```python
from build123d import *

# Parameters (mm, degrees)
SKETCH1_R           = 10.5
BOSS_EXTRUDE1_DEPTH = 16.5
SKETCH2_R           = 7.5
CUT_EXTRUDE1_DEPTH  = 9
SKETCH15_R          = 0.5
CUT_EXTRUDE10_DEPTH = 3
CIRPATTERN1_COUNT   = 4
SKETCH11_R          = 2.75
CUT_EXTRUDE6_DEPTH  = 23.19797288
SKETCH13_W          = 5
SKETCH13_H          = 21
CUT_EXTRUDE8_DEPTH  = 23.197973064
SKETCH14_R          = 0.5
CUT_EXTRUDE9_DEPTH  = 2


with BuildPart() as part:
    # Sketch1 → Boss-Extrude1 (new body)
    with BuildSketch(Plane.XY):
        Circle(SKETCH1_R)
    extrude(amount=BOSS_EXTRUDE1_DEPTH)

    # Sketch2 → Cut-Extrude1 (cut)
    with BuildSketch(Plane.XY.offset(16.5)):
        Circle(SKETCH2_R)
    extrude(amount=-CUT_EXTRUDE1_DEPTH, mode=Mode.SUBTRACT)

    # Sketch15 → Cut-Extrude10 (cut)
    with BuildSketch(Plane.XY.offset(16.5)):
        with Locations((6.363961031, 6.363961031)):
            Circle(SKETCH15_R)
    cut_extrude10 = extrude(amount=-CUT_EXTRUDE10_DEPTH, mode=Mode.SUBTRACT)

    # CirPattern1: Cut-Extrude10 ×4 about axis
    cirpattern1_axis = Axis((0, 0, 0), (0, 0, 1))
    for i in range(1, CIRPATTERN1_COUNT):
        add(cut_extrude10.rotate(cirpattern1_axis, i * 360 / CIRPATTERN1_COUNT), mode=Mode.SUBTRACT)

    # Sketch9 → Cut-Revolve1 (revolve, cut)
    with BuildSketch(Plane(origin=(0, 0, 0), x_dir=(0, 0, -1), z_dir=(1, 0, 0)), mode=Mode.PRIVATE) as cut_revolve1_sk:
        Polygon((-5, 0), (-5, 7.5), (-2.5, 7.5), (-2.5, 5.5), (0, 5.5), (0, 0), align=None)
    revolve(cut_revolve1_sk.sketch.rotate(Axis((0, 0, 0), (0, 0, 1)), 90), axis=Axis((0, 0, 0), (0, 0, 1)), mode=Mode.SUBTRACT)

    # Sketch11 → Cut-Extrude6 (cut, through all)
    with BuildSketch(Plane(origin=(0, 0, 0), x_dir=(0, 0, -1), z_dir=(1, 0, 0))):
        with Locations((-11.75, 0)):
            Circle(SKETCH11_R)
    extrude(amount=-CUT_EXTRUDE6_DEPTH, mode=Mode.SUBTRACT)

    # Sketch13 → Cut-Extrude8 (cut, through all)
    with BuildSketch(Plane(origin=(0, 0, 0), x_dir=(0, 0, -1), z_dir=(1, 0, 0))):
        with Locations((-2.5, 0)):
            Rectangle(SKETCH13_W, SKETCH13_H)
    extrude(amount=-CUT_EXTRUDE8_DEPTH, mode=Mode.SUBTRACT)

    # Sketch14 → Cut-Extrude9 (cut)
    with BuildSketch(Plane.ZY):
        with Locations((2.5, 9)):
            Circle(SKETCH14_R)
    cut_extrude9 = extrude(amount=-CUT_EXTRUDE9_DEPTH, mode=Mode.SUBTRACT)

    # Mirror1: Cut-Extrude9 across plane
    add(cut_extrude9.mirror(Plane.ZX), mode=Mode.SUBTRACT)


solid = part.part
```
Geometry: final body of the model. Coordinates: model frame, mm. A direction names the side the tool comes from. Round coordinates to 2 decimals unless told otherwise and drop trailing zeros. Order: outer loops, then holes, each group sorted by start corner. A loop starts at its lowest first (then second) coordinate and runs counter-clockwise, first axis right, second up. Notation, with made-up numbers: (-4.75, 26) -> (4.25, 26) arc R24 cw to (4.25, 59) -> close; hole circle Ø5 at (42.25, -1). An arc over 180 degrees is marked (long way). Use one line per item in the form item = value.
(1) Access query for faces 4 (the face through (2, -9, 2.5)), 5 (the face through (0, 8.59, 1.98)), 6 (the face through (5, -7, 16.5)), 7 (the face through (6, 0, 0)), 8 (the face through (6.4, -6.4, 13.5)). Directions: +Z, -Z, +X, -X, +Y, -Y. A direction counts if a zero-diameter tool reaches every point of the face in a straight line with its end or side. Return the directions, or none.
Results list:
face_4 = -X
face_5 = -Z, -X, +Y, -Y
face_6 = +Z, +X, -X, +Y, -Y
face_7 = -Z, +X, -X, +Y, -Y
face_8 = +Z
(2) First-contact query: pin 1 Ø3 at (y, z) = (-6.5, 5.5) entering from -X; pin 2 Ø1 at (x, z) = (-3.5, 14) entering from -Y; pin 3 Ø0.5 at (y, z) = (9, 2.5) entering from -X. Flat tips, straight axial feed; report the tip coordinate or a pass-through.
Results list:
pin_1 = -9.23
pin_2 = -10.06
pin_3 = 2
(3) Draft query along Z for faces 1 (the face through (1, -9, 2)), 2 (the face through (-6.4, 6.4, 13.5)), 3 (the face through (6.841, 6.514, 15.021)). Return one class per face: pulls with the +Z half, pulls with the -Z half, needs draft (parallel to the pull), parting line crosses it, or undercut.
Results list:
face_1 = undercut
face_2 = pulls with the +Z half
face_3 = needs draft
(4) Section D-D on z = 5.5. Return loops of the section in (x, y), and give its area (3 significant figures).
Results list:
outline = circle Ø21 at (0, 0)
area = 346 mm^2
(5) Section B-B on x = 1.5. Return loops of the section in (y, z), and give its area (3 significant figures).
Results list:
outline = (-10.39, 0) -> (-5.29, 0) -> (-5.29, 2.5) -> (-7.35, 2.5) -> (-7.35, 5) -> (7.35, 5) -> (7.35, 2.5) -> (5.29, 2.5) -> (5.29, 0) -> (10.39, 0) -> (10.39, 16.5) -> (7.35, 16.5) -> (7.35, 7.5) -> (-7.35, 7.5) -> (-7.35, 16.5) -> (-10.39, 16.5) -> close; hole circle Ø1 at (-9, 2.5); hole circle Ø1 at (9, 2.5)
area = 146 mm^2
(6) Ray query, probe 1 along Z at (x, y) = (6.25, -4); probe 2 along Z at (x, y) = (0.95, -9); probe 3 along Z at (x, y) = (-4.25, -0.5). Return the intervals inside material, ascending. Write a range as [from, to].
Results list:
probe_1 = [0, 2.5], [5, 7.5]
probe_2 = [0, 2], [3, 16.5]
probe_3 = [5, 7.5]
(7) Section A-A on y = 0. Return loops of the section in (x, z).
Results list:
outline = (-10.5, 5) -> (7.5, 5) -> (7.5, 2.5) -> (5.5, 2.5) -> (5.5, 0) -> (10.5, 0) -> (10.5, 16.5) -> (7.5, 16.5) -> (7.5, 7.5) -> (-7.5, 7.5) -> (-7.5, 9) -> (-10.5, 9) -> close; (-10.5, 14.5) -> (-7.5, 14.5) -> (-7.5, 16.5) -> (-10.5, 16.5) -> close
(8) Section C-C on x = -8.5. Return loops of the section in (y, z), and give its area (3 significant figures).
Results list:
outline = (-6.16, 5) -> (6.16, 5) -> (6.16, 16.5) -> (-6.16, 16.5) -> close; hole circle Ø5.5 at (0, 11.75)
area = 118 mm^2
